Part model, mm, in its own coordinate system. Face numbers are marked on the shaded views. Round coordinates to 2 decimals unless told otherwise and drop trailing zeros. Write each loop counter-clockwise with the first axis right and the second up, starting at its lowest first coordinate (ties: lowest second). Pieces come first, ordered by that corner, then holes. Notation, with made-up numbers: (42.25, -5) -> (61.25, -5) arc R25 cw to (61.25, 13) -> close; hole circle Ø11 at (9, 26). An arc over 180 degrees is marked (long way). Return JSON: item names as keys, results as strings. Group by question number.
(1) Drill centre lines: L1, parallel to Y at x = 75.5, z = 8 (3 decimals); L2, parallel to X at y = -94, z = 7.75 (3 decimals); L3, parallel to Z at x = 78.5, y = -73.5. Where is each one in solid material? Low to high. Write a range as from..to.
(2) Drop a flat-ended pin along its axis: pin 1 Ø6 at (x, y) = (72.5, -31.5) entering from +Z. Give the stop position or say it passes through.
(3) Mould opens along Y. For the marked faces 1 and 2 say: +Y half, -Y half, draft (parallel to the pull), parting line (faces both ways), or undercut.
(4) Saw through at A-A (y = -28). List the corners of the cut face in (x, z) (3 decimals), plus the area to 3 significant figures.
(5) Saw through at C-C (y = -68.5). List the corners of the cut face in (x, z) (3 decimals), plus the area to 3 significant figures.
(6) Saw through at B-B (x = 113). List the corners of the cut face in (y, z) (3 decimals), plus the area to 3 significant figures.
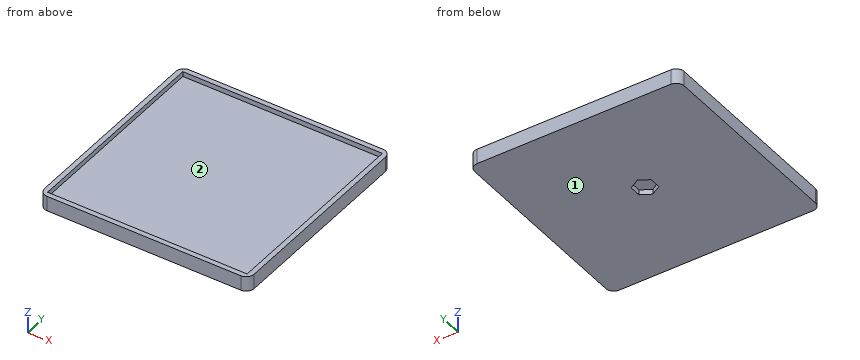
from build123d import *

# Parameters (mm, degrees)
F0_W     = 133.35
F0_H     = 133.35
F1_DEPTH = 6.35
F2_W     = 133.35
F2_H     = 133.35
F2_W_2   = 127
F2_H_2   = 127
F3_DEPTH = 3.175
F6_DEPTH = 3.175
F7_R     = 5.08


with BuildPart() as f1:
    # F0 (on Top) → F1 (new body)
    with BuildSketch(Plane.XY):
        with Locations((66.675, -66.675)):
            Rectangle(F0_W, F0_H)
    extrude(amount=F1_DEPTH)

    # F2 (on face) → F3 (join)
    with BuildSketch(Plane.XY.offset(6.35)):
        with Locations((66.675, -66.675)):
            Rectangle(F2_W, F2_H)
        with Locations((66.675, -66.675)):
            Rectangle(F2_W_2, F2_H_2, mode=Mode.SUBTRACT)
    extrude(amount=F3_DEPTH)

    # F5 (on face) → F6 (cut)
    with BuildSketch(Plane(origin=(0, 0, 0), x_dir=(1, 0, 0), z_dir=(0, 0, -1))):
        Polygon((73.025, 63.008826), (73.025, 70.341174), (66.675, 74.007348), (60.325, 70.341174), (60.325, 63.008826), (66.675, 59.342652), align=None)
    extrude(amount=-F6_DEPTH, mode=Mode.SUBTRACT)

    # F7
    f7_edges = [f1.edges().sort_by_distance(p)[0] for p in [
        (133.35, -133.35, 4.7625),
        (133.35, 0, 4.7625),
        (0, 0, 4.7625),
        (0, -133.35, 4.7625),
    ]]
    fillet(f7_edges, radius=F7_R)


solid = f1.part
Computed values:
{
 "1": {"L1": "-133.35..-130.175, -3.175..0", "L2": "0..3.175, 130.175..133.35", "L3": "0..6.35"},
 "2": {"pin 1": "z = 6.35"},
 "3": {"face 1": "draft", "face 2": "undercut"},
 "4": {"outline": "(0, 0) -> (133.35, 0) -> (133.35, 9.525) -> (130.175, 9.525) -> (130.175, 6.35) -> (3.175, 6.35) -> (3.175, 9.525) -> (0, 9.525) -> close", "area": "867 mm2"},
 "5": {"outline": "(0, 0) -> (60.325, 0) -> (60.325, 3.175) -> (73.025, 3.175) -> (73.025, 0) -> (133.35, 0) -> (133.35, 9.525) -> (130.175, 9.525) -> (130.175, 6.35) -> (3.175, 6.35) -> (3.175, 9.525) -> (0, 9.525) -> close", "area": "827 mm2"},
 "6": {"outline": "(-133.35, 0) -> (0, 0) -> (0, 9.525) -> (-3.175, 9.525) -> (-3.175, 6.35) -> (-130.175, 6.35) -> (-130.175, 9.525) -> (-133.35, 9.525) -> close", "area": "867 mm2"}
}
